Check sheet for the drawn part. Datum: minimum x, y, z corner. Units: mm. A direction names the side the tool comes from. Round coordinates to 2 decimals unless told otherwise and drop trailing zeros. Write each loop counter-clockwise with the first axis right and the second up, starting at its lowest first coordinate (ties: lowest second). Pieces come first, ordered by that corner, then holes. Notation, with made-up numbers: M -20,-18 L 9,-18 A35 ccw 9,17 Z; hole C 44.5,-17 d4. An arc over 180 degrees is marked long. One line per item, written item: value.
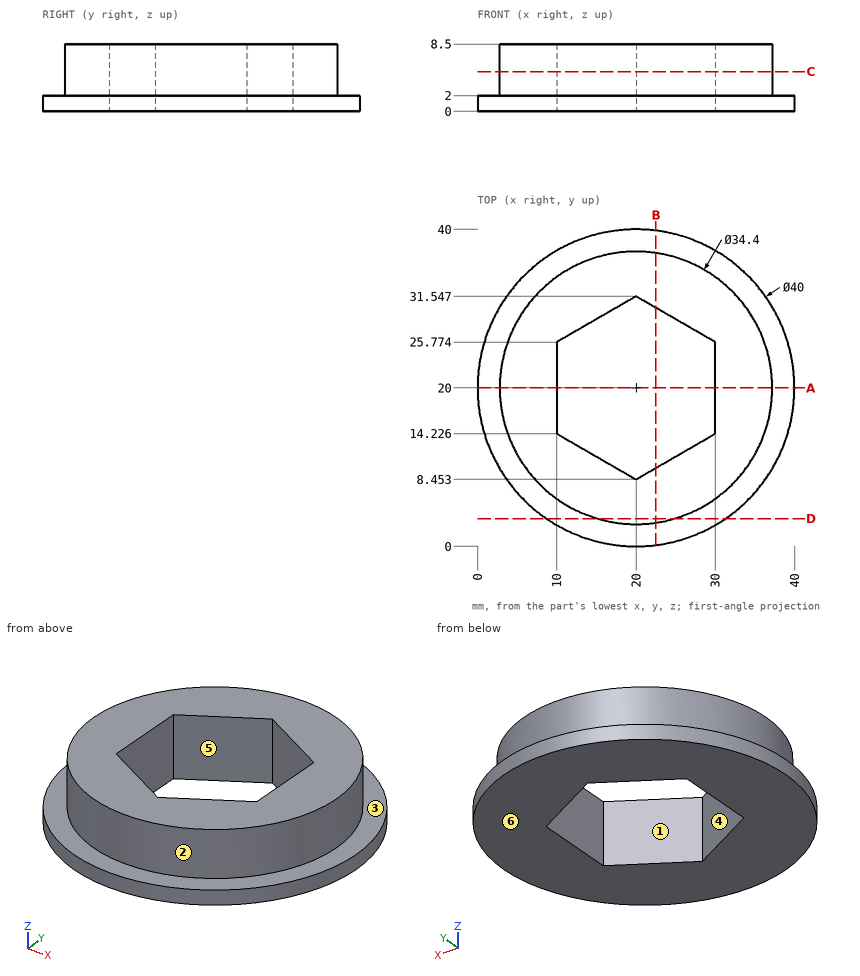
Q1. Depth check by flat-ended pin: P1, Ø4, axis at y = 18, z = 5, coming from the -X side; P2, Ø3, axis at x = 27.5, z = 1.5, coming from the -Y side; P3, Ø1.5, axis at x = 28.5, y = 25, coming from the +Z side; P4, Ø12, axis at x = 15, y = 29, coming from the -Z side. Enter the tip coordinate at first touch or a pass-through.
Completed:
P1: x = 2.8
P2: y = 0.92
P3: through
P4: z = 0
Q2. Sectioned sample at D-D on y = 3.5. Enter the section's corners in (x, z).
Completed:
outline: M 8.7,0 L 31.3,0 L 31.3,2 L 24.86,2 L 24.86,8.5 L 15.14,8.5 L 15.14,2 L 8.7,2 Z
Q3. Access from +Z, -Z, +X, -X, +Y, -Y to the whole of each face (thin tool, end or side, straight path). Record for the marked faces 5 and 6.
Completed:
face 5: +Z, -Z
face 6: -Z, +X, -X, +Y, -Y
Q4. Sectioned sample at A-A on y = 20. Enter the section's corners in (x, z), and give its area (3 significant figures).
Completed:
outline: M 0,0 L 10,0 L 10,8.5 L 2.8,8.5 L 2.8,2 L 0,2 Z; M 30,0 L 40,0 L 40,2 L 37.2,2 L 37.2,8.5 L 30,8.5 Z
area: 134 mm^2
Q5. Sectioned sample at C-C on z = 5. Enter the section's corners in (x, y).
Completed:
outline: C 20,20 d34.4; hole M 10,14.23 L 20,8.45 L 30,14.23 L 30,25.77 L 20,31.55 L 10,25.77 Z
Q6. Scan lines: line 1 (X direction, y = 20.5, z = 4); line 2 (Y direction, x = 17, z = 5.75) (1 decimal); line 3 (X direction, y = 8.5, z = 3.5) (1 decimal). Record each from-to range of solid material in increasing order. Write a range as [from, to].
Completed:
line 1: [2.81, 10], [30, 37.19]
line 2: [3.1, 10.2], [29.8, 36.9]
line 3: [7.2, 19.9], [20.1, 32.8]
Q7. Sectioned sample at B-B on x = 22.5. Enter the section's corners in (y, z).
Completed:
outline: M 0.16,0 L 9.9,0 L 9.9,8.5 L 2.98,8.5 L 2.98,2 L 0.16,2 Z; M 30.1,0 L 39.84,0 L 39.84,2 L 37.02,2 L 37.02,8.5 L 30.1,8.5 Z
Q8. Draft check along Y on the marked faces 1, 2, 3 and 4. Enter one of: pulls with the +Y half, pulls with the -Y half, needs draft (parallel to the pull), parting line crosses it, or undercut.
Completed:
face 1: undercut
face 2: parting line crosses it
face 3: needs draft
face 4: undercut
